Read the model definition and answer for the solid it produces. Units are mm, in the model's axes. A direction names the side the tool comes from. Give positions to 0.01 mm unless a question says otherwise; leave off trailing zeros. Order: outer loops, then holes, each group sorted by start corner. A loop starts at its lowest first (then second) coordinate and runs counter-clockwise, first axis right, second up. Notation, with made-up numbers: (23.25, -1) -> (60.25, -1) arc R31 cw to (60.25, 28) -> close; hole circle Ø1 at (12, 89.5). An arc over 180 degrees is marked (long way). Use one line per item in the form item = value.
```python
from build123d import *

# Parameters (mm, degrees)
F1_DEPTH = 25.4
F2_DEPTH = 50.8
F4_R     = 7.355255
F5_DEPTH = 62.131667


with BuildPart() as f1:
    # F0 (on Front) → F1 (new body)
    with BuildSketch(Plane.XZ):
        with BuildLine():
            Line((-62.279664, 0), (-62.279664, -62.130667))
            Line((-62.279664, -62.130667), (62.279664, -62.130667))
            Line((62.279664, -62.130667), (62.279664, 0))
            Line((62.279664, 0), (33.608398, 0))
            ThreePointArc((33.608398, 0), (0, -33.608398), (-33.608398, 0))
            Line((-33.608398, 0), (-62.279664, 0))
        make_face()
        with BuildLine():
            Line((-18.182814, 0), (-33.608398, 0))
            ThreePointArc((-33.608398, 0), (0, -33.608398), (33.608398, 0))
            Line((33.608398, 0), (18.182814, 0))
            ThreePointArc((18.182814, 0), (0, -18.182814), (-18.182814, 0))
        make_face()
    extrude(amount=F1_DEPTH)

    # F0 (on Front) → F2 (join)
    with BuildSketch(Plane.XZ):
        with BuildLine():
            Line((-18.182814, 0), (-33.608398, 0))
            ThreePointArc((-33.608398, 0), (0, -33.608398), (33.608398, 0))
            Line((33.608398, 0), (18.182814, 0))
            ThreePointArc((18.182814, 0), (0, -18.182814), (-18.182814, 0))
        make_face()
    extrude(amount=F2_DEPTH)

    # F3: F1 across plane


with BuildPart() as f1_1:
    add(f1.part)
    add(f1.part.mirror(Plane.XZ))

    # F4 (on face) → F5 (cut, through all)
    with BuildSketch(Plane.XY):
        with Locations((-47.380224, 0)):
            Circle(F4_R)
        with Locations((47.380224, 0)):
            Circle(F4_R)
    extrude(amount=-F5_DEPTH, mode=Mode.SUBTRACT)


solid = f1_1.part
```
Item 1: Which of the six approach directions +Z, -Z, +X, -X, +Y, -Y give full straight-line access (tool end or side, diameter ignored) to faces 4 (the flat face through (-1, -25.4, -38)), 5 (the flat face through (36, -1, 0)), 6 (the cylindrical face through (-0.7, 37.9, -33.6))?
Checks:
face_4 = -Z, -Y
face_5 = +Z, +X, -X, +Y, -Y
face_6 = -Z, +Y
Item 2: The part is cut by section A-A on y = 0. Give the vertices of the cut face in (x, z).
Checks:
outline = (-62.28, -62.13) -> (-54.74, -62.13) -> (-54.74, 0) -> (-62.28, 0) -> close; (-40.02, -62.13) -> (40.02, -62.13) -> (40.02, 0) -> (18.18, 0) arc R18.18 cw to (-18.18, 0) -> (-40.02, 0) -> close; (54.74, -62.13) -> (62.28, -62.13) -> (62.28, 0) -> (54.74, 0) -> close
Item 3: The part is cut by section C-C on x = -42. Give the vertices of the cut face in (y, z), and give its area (3 significant figures).
Checks:
outline = (-25.4, -62.13) -> (-5.02, -62.13) -> (-5.02, 0) -> (-25.4, 0) -> close; (5.02, -62.13) -> (25.4, -62.13) -> (25.4, 0) -> (5.02, 0) -> close
area = 2,530 mm²
Item 4: The part is cut by section D-D on x = 0. Give the vertices of the cut face in (y, z).
Checks:
outline = (-50.8, -33.61) -> (-25.4, -33.61) -> (-25.4, -62.13) -> (25.4, -62.13) -> (25.4, -33.61) -> (50.8, -33.61) -> (50.8, -18.18) -> (-50.8, -18.18) -> close
Item 5: Determine the mould class of faces 1 (the flat face through (-62.28, 0, -31)), 2 (the flat face through (0, 50.8, -20)), 3 (the cylindrical face through (0.4, -0.71, -18.18)) for opening direction X: +X half, -X half, draft (parallel to the pull), parting line (faces both ways), or undercut.
Checks:
face_1 = -X half
face_2 = draft
face_3 = undercut
Item 6: Straight lines are drawn through the part: L1, parallel to X at y = -4.5, z = -9.5; L2, parallel to Y at x = -4.5, z = -36.5; L3, parallel to X at y = 15.5, z = -4. For each, find the intervals that lie inside material, in ascending order. Write a range as from..to.
Checks:
L1 = -62.28..-53.2, -41.56..-15.5, 15.5..41.56, 53.2..62.28
L2 = -25.4..25.4
L3 = -62.28..-17.74, 17.74..62.28
Item 7: Given pin 1 Ø10 at (x, z) = (35, -23.5) entering from -Y; pin 2 Ø5 at (x, z) = (19.5, -54.5) entering from +Y, each flat-ended and moving along its own axis, determine where each tip first touches the part or whether it passes through.
Checks:
pin_1 = -25.4
pin_2 = 25.4
Item 8: The part is cut by section B-B on z = -6. Give the vertices of the cut face in (x, y), and give its area (3 significant figures).
Checks:
outline = (-62.28, -25.4) -> (-33.07, -25.4) -> (-33.07, -50.8) -> (-17.16, -50.8) -> (-17.16, 50.8) -> (-33.07, 50.8) -> (-33.07, 25.4) -> (-62.28, 25.4) -> close; (17.16, -50.8) -> (33.07, -50.8) -> (33.07, -25.4) -> (62.28, -25.4) -> (62.28, 25.4) -> (33.07, 25.4) -> (33.07, 50.8) -> (17.16, 50.8) -> close; hole circle Ø14.71 at (-47.38, 0); hole circle Ø14.71 at (47.38, 0)
area = 5,860 mm²
